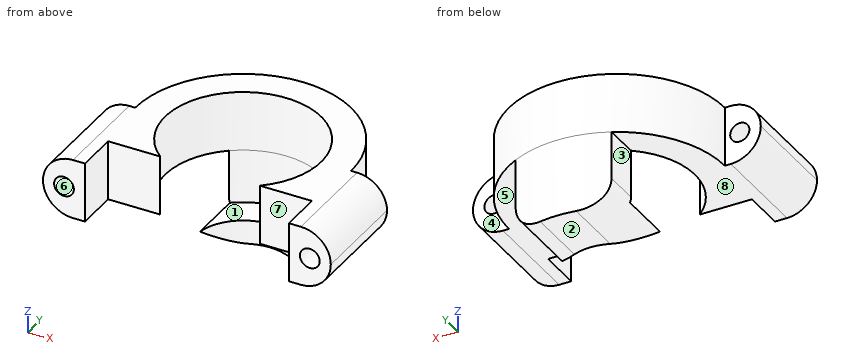
```python
from build123d import *
from build123d.topology import SkipClean

# Parameters (mm, degrees)
SKETCH1_R             = 6
EXTRUDE1_DEPTH        = 10
SKETCH2_R             = 13
CUT_EXTRUDE1_DEPTH    = 6
SKETCH3_R             = 1.6
CUT_EXTRUDE2_DEPTH    = 10
SKETCH4_W             = 7
SKETCH4_H             = 10
SKETCH4_R             = 1.6
EXTRUDE3_DEPTH        = 7
FILLET2_R             = 5
SKETCH5_R             = 13
EXTRUDE4_DEPTH        = 4
EXTRUDE5_START        = 9
EXTRUDE5_DEPTH        = 9
EXTRUDE6_START        = 4
EXTRUDE6_DEPTH        = 4
FILLET3_R             = 5
M4_TAPPED_HOLE1_D     = 3.3
M4_TAPPED_HOLE1_DEPTH = 10.1
M4_TAPPED_HOLE1_TIP   = 0.991420021


# Some blends are built 0.0001 mm under size
with BuildPart() as part:
    # Sketch1 → Extrude1 (new body)
    with BuildSketch(Plane.XY):
        with BuildLine():
            Line((-18, 0), (-24, 0))
            Line((-24, 0), (-24, -10))
            Line((-24, -10), (24, -10))
            Line((24, -10), (24, 0))
            Line((24, 0), (18, 0))
            ThreePointArc((18, 0), (0, 18.000000653), (-18, 0))
        make_face()
        with Locations((0, 6.53e-07)):
            Circle(SKETCH1_R, mode=Mode.SUBTRACT)
    extrude(amount=EXTRUDE1_DEPTH)

    # Sketch2 → Cut-Extrude1 (cut)
    with BuildSketch(Plane(origin=(0, 0, 0), x_dir=(-1, 0, 0), z_dir=(0, 0, -1))):
        Circle(SKETCH2_R)
    extrude(amount=-CUT_EXTRUDE1_DEPTH, mode=Mode.SUBTRACT)

    # Sketch3 → Cut-Extrude2 (cut)
    with BuildSketch(Plane(origin=(0, 0, 0), x_dir=(-1, 0, 0), z_dir=(0, 1, 0))):
        with Locations(Location((-20.5, 5, 0), (0, 0, 90))):
            Circle(SKETCH3_R)
        with Locations(Location((20.5, 5, 0), (0, 0, 90))):
            Circle(SKETCH3_R)
    extrude(amount=-CUT_EXTRUDE2_DEPTH, mode=Mode.SUBTRACT)

    # Sketch4 → Extrude3 (add)
    # profile 1 of 2: a face of its own
    with SkipClean():  # the faces are left unmerged after this step: merging them gives an invalid solid
        with BuildSketch(Plane.XZ.offset(10)):
            with Locations((-20.5, 5)):
                Rectangle(SKETCH4_W, SKETCH4_H)
            with Locations((-20.5, 5)):
                Circle(SKETCH4_R, mode=Mode.SUBTRACT)
        # profile 2 of 2: a face of its own
        with BuildSketch(Plane.XZ.offset(10)):
            with Locations((20.5, 5)):
                Rectangle(SKETCH4_W, SKETCH4_H)
            with Locations((20.5, 5)):
                Circle(SKETCH4_R, mode=Mode.SUBTRACT)
        extrude(amount=EXTRUDE3_DEPTH)
    add(part.part.scale(1), mode=Mode.REPLACE)  # the faces are merged on a copy

    # Fillet2
    fillet2_edges = [part.edges().sort_by_distance(p)[0] for p in [
        (24, -8.5, 10),
        (24, -8.5, 0),
        (-24, -5, 10),
        (-24, -5, 0),
    ]]
    fillet(fillet2_edges, radius=FILLET2_R - 0.0001)  # a hair under: the kernel refuses the full size

    # Sketch5 → Extrude4 (cut)
    with BuildSketch(Plane(origin=(0, 0, 6), x_dir=(-1, 0, 0), z_dir=(0, 0, -1))):
        Circle(SKETCH5_R)
    extrude(amount=-EXTRUDE4_DEPTH, mode=Mode.SUBTRACT)

    # Sketch6 → Extrude5 (add)
    with BuildSketch(Plane(origin=(0, 0, 0), x_dir=(-1, 0, 0), z_dir=(0, 0, -1)).offset(EXTRUDE5_START)):
        with BuildLine():
            Line((-8, 10.246950766), (-8, 16.12451615))
            ThreePointArc((-8, 16.12451615), (0, 18.000000585), (8, 16.12451615))
            Line((8, 16.12451615), (8, 10.246950766))
            ThreePointArc((8, 10.246950766), (0, 13), (-8, 10.246950766))
        make_face()
    extrude(amount=-EXTRUDE5_DEPTH)

    # Sketch7 → Extrude6 (add)
    with BuildSketch(Plane(origin=(0, 0, -9), x_dir=(-1, 0, 0), z_dir=(0, 0, -1)).offset(EXTRUDE6_START)):
        with BuildLine():
            Line((8, 16.12451615), (8, 0))
            ThreePointArc((8, 0), (0, 8), (-8, 0))
            Line((-8, 0), (-8, 16.12451615))
            ThreePointArc((-8, 16.12451615), (0, 18.000000585), (8, 16.12451615))
        make_face()
    extrude(amount=-EXTRUDE6_DEPTH)

    # Fillet3
    # the kernel refuses this fillet: 5 mm, written as the material it takes off along each edge
    with BuildSketch(Plane(origin=(-8, 28.62451615, -13), x_dir=(0, 0, 1), z_dir=(0, -1, 0)), Plane(origin=(8, -12.5, -13), x_dir=(0, 0, 1), z_dir=(0, 1, 0))) as fillet3_piece_1:
        with BuildLine():
            CenterArc((FILLET3_R, -FILLET3_R), FILLET3_R, 90, 90)
            Line((0, -FILLET3_R), (0, 0))
            Line((0, 0), (FILLET3_R, 0))
        make_face()
    extrude(amount=41.12451615, mode=Mode.SUBTRACT)

    # M4 Tapped Hole1
    with Locations(Plane(origin=(-20.5, -17, 5), x_dir=(0, 0, -1), z_dir=(0, -1, 0))):
        with Locations((0, 0), (0, 41)):
            Hole(M4_TAPPED_HOLE1_D / 2, depth=M4_TAPPED_HOLE1_DEPTH)
            with Locations((0, 0, -(M4_TAPPED_HOLE1_DEPTH + M4_TAPPED_HOLE1_TIP / 2))):  # 118° drill point
                Cone(0, M4_TAPPED_HOLE1_D / 2, M4_TAPPED_HOLE1_TIP, mode=Mode.SUBTRACT)


solid = part.part
```
Can you work these out from the model? Positions are in its coordinate system, mm. Face numbers are marked on the shaded views. A direction names the side the tool comes from. Coordinates: 2 decimals unless noted, no trailing zeros. Order: outer loops, then holes, each group sorted by start corner. A loop starts at its lowest first (then second) coordinate and runs counter-clockwise, first axis right, second up.
1. If we section it at A-A (y = -15): Give the number of separate pieces and of enclosed holes in the cut face, then the cut area to 3 significant figures.
2. I need wall thicknesses on line 1 (X direction, y = -12, z = 5); line 2 (Y direction, x = 18.5, z = 8.5); line 3 (X direction, y = -2, z = 5). Which ranges of each line are inside material? Lowest first, please.
3. Thinking about a two-plate mould opening in X: for the marked faces 1, 2 and 3, which applies, +X half, -X half, draft (parallel to the pull), parting line (faces both ways), or undercut?
4. If we section it at C-C (x = 20.5): Please give me the cut outline in (y, z), then the cut area to 3 significant figures.
5. I'm going to push flat-ended pins straight in: pin 1 (9 mm diameter, centred on x = -16, y = -8.5, fed in from -Z); pin 2 (2.5 mm diameter, centred on x = -11, z = 4.5, fed in from -Y); pin 3 (5 mm diameter, centred on x = 21.5, z = 5.5, fed in from +Y). Where does each tip first touch, or does it pass through?
6. For the marked faces 4, 5, 6, 7 and 8, which set-ups out of +Z, -Z, +X, -X, +Y, -Y let a thin tool reach every point of the face, with its end or its side?
7. If we section it at B-B (y = 2): Please give me the cut outline in (x, z).
Entries:
1. separate pieces: 2
1. enclosed holes: 2
1. area: 101 mm2
2. line 1: x = -24 to -22.15, -18.85 to -17, 17 to 18.85, 22.15 to 24
2. line 2: y = -17 to 0
2. line 3: x = -24 to -22.1, -18.9 to -12.85, 12.85 to 18.9, 22.1 to 24
3. face 1: undercut
3. face 2: draft
3. face 3: -X half
4. outline: (-17, 0.23) - (0, 0.23) - (0, 3.4) - (-6.87, 3.4) - (-6.9, 3.35) - (-17, 3.35) - close; (-17, 6.65) - (-6.9, 6.65) - (-6.87, 6.6) - (0, 6.6) - (0, 9.77) - (-17, 9.77) - close
4. area: 107 mm2
5. pin 1: stops at z = 0
5. pin 2: stops at y = -10
5. pin 3: stops at y = 0
6. face 4: +Z, -Z, +X, +Y
6. face 5: -Z, +X, +Y, -Y
6. face 6: -Y
6. face 7: +Z, -Z, -Y
6. face 8: -Z, -X, +Y, -Y
7. outline: (-17.89, 0) - (-12.85, 0) - (-12.85, 10) - (-17.89, 10) - close; (-7.9, -9) arc R5 ccw to (-7.75, -9.57) - (-7.75, -9) - close; (7.75, -9.57) arc R5 ccw to (7.9, -9) - (7.75, -9) - close; (12.85, 0) - (17.89, 0) - (17.89, 10) - (12.85, 10) - close
